from build123d import *

# Parameters (mm, degrees)
SKETCH1_W            = 81.28
SKETCH1_H            = 81.28
SKETCH1_W_2          = 76.2
SKETCH1_H_2          = 76.2
BOSS_EXTRUDE1_DEPTH  = 177.8
SKETCH2_W            = 2.54
SKETCH2_H            = 38.1
BOSS_EXTRUDE2_DEPTH  = 25.4
SKETCH3_W            = 2.54
SKETCH3_H            = 25.4
CUT_EXTRUDE1_DEPTH   = 212.720846399
BOSS_EXTRUDE3_DEPTH  = 12.7
BOSS_EXTRUDE4_DEPTH  = 12.7
SKETCH14_W           = 5.08
SKETCH14_H           = 25.4
BOSS_EXTRUDE6_DEPTH  = 76.2
CUT_EXTRUDE2_REACH   = 243.407
SKETCH16_W           = 23.13
SKETCH16_H           = 20.32
SKETCH22_R           = 2
CUT_EXTRUDE6_DEPTH   = 252.036309724
SKETCH28_W           = 35.399999812
SKETCH28_H           = 50.8
BOSS_EXTRUDE7_DEPTH  = 38.1
CUT_EXTRUDE8_REACH   = 246.574
SKETCH32_W           = 33.02
SKETCH32_H           = 30.319999812
CUT_EXTRUDE9_DEPTH   = 25.4
CUT_EXTRUDE13_REACH  = 245.27
SKETCH34_R           = 9.890000016
BOSS_EXTRUDE9_DEPTH  = 2.54
SKETCH38_W           = 2.54
SKETCH38_H           = 25.4
CUT_EXTRUDE15_DEPTH  = 63.5
CUT_EXTRUDE17_REACH  = 224.71
SKETCH40_R           = 2.999995
SKETCH41_R           = 3.77
SKETCH41_R_2         = 2.5
BOSS_EXTRUDE10_DEPTH = 5
BOSS_EXTRUDE11_START = 5
SKETCH42_R           = 3.77
SKETCH42_R_2         = 2.5
BOSS_EXTRUDE11_DEPTH = 5
SKETCH43_W           = 76.2
SKETCH43_H           = 76.2
CUT_EXTRUDE20_DEPTH  = 25.4
SKETCH44_W           = 174.6
SKETCH44_H           = 70
SKETCH44_R           = 1.5
BOSS_EXTRUDE12_DEPTH = 2.54
FILLET1_R            = 5.08
FILLET2_R            = 12.7
FILLET3_R            = 2.54
FILLET7_R            = 12.7
FILLET9_R            = 12.7
BOSS_EXTRUDE20_DEPTH = 88.9
CUT_EXTRUDE21_REACH  = 275.109
SKETCH54_R           = 2.5
FILLET11_R           = 2.54
FILLET12_R           = 2.54


with BuildPart() as part:
    # Sketch1 → Boss-Extrude1 (new body)
    with BuildSketch(Plane(origin=(0, 0, 0), x_dir=(1, 0, 0), z_dir=(0, 1, 0))):
        with Locations((40.64, 40.64)):
            Rectangle(SKETCH1_W, SKETCH1_H)
        with Locations((40.64, 40.64)):
            Rectangle(SKETCH1_W_2, SKETCH1_H_2, mode=Mode.SUBTRACT)
    extrude(amount=BOSS_EXTRUDE1_DEPTH)

    # Sketch2 → Boss-Extrude2 (add)
    with BuildSketch(Plane(origin=(0, 0, 0), x_dir=(0, 0, -1), z_dir=(1, 0, 0))):
        with Locations((64.77, 19.05)):
            Rectangle(SKETCH2_W, SKETCH2_H)
    extrude(amount=-BOSS_EXTRUDE2_DEPTH)

    # Sketch3 → Cut-Extrude1 (cut, through all)
    with BuildSketch(Plane.XY):
        with Locations((80.01, 12.7)):
            Rectangle(SKETCH3_W, SKETCH3_H)
    extrude(amount=-CUT_EXTRUDE1_DEPTH, mode=Mode.SUBTRACT)

    # Sketch7 → Boss-Extrude3 (add)
    with BuildSketch(Plane.XY):
        Polygon((81.28, 25.4), (106.68, 50.8), (81.28, 50.8), align=None)
    extrude(amount=-BOSS_EXTRUDE3_DEPTH)

    # Sketch10 → Boss-Extrude4 (add)
    with BuildSketch(Plane(origin=(0, 0, -81.28), x_dir=(-1, 0, 0), z_dir=(0, 0, -1))):
        Polygon((-81.28, 25.4), (-81.28, 50.8), (-106.68, 50.8), align=None)
    extrude(amount=-BOSS_EXTRUDE4_DEPTH)

    # Sketch14 → Boss-Extrude6 (add)
    with BuildSketch(Plane(origin=(81.28, 0, 0), x_dir=(0, 0, -1), z_dir=(1, 0, 0))):
        with Locations((40.64, 38.1)):
            Rectangle(SKETCH14_W, SKETCH14_H)
    extrude(amount=BOSS_EXTRUDE6_DEPTH)

    # Sketch16 → Cut-Extrude2 (cut, up to next)
    with BuildSketch(Plane.XY.offset(-38.1), mode=Mode.PRIVATE) as cut_extrude2_sk1:
        with Locations((129.405, 40.64)):
            Rectangle(SKETCH16_W, SKETCH16_H)
    cut_extrude2_tool1 = extrude(cut_extrude2_sk1.sketch, amount=-CUT_EXTRUDE2_REACH, mode=Mode.PRIVATE) & part.part
    add(cut_extrude2_tool1.solids().sort_by_distance((129.405, 40.64, -38.1))[0], mode=Mode.SUBTRACT)

    # Sketch22 → Cut-Extrude6 (cut, through all)
    with BuildSketch(Plane.XY):
        with Locations((93.98, 45.72)):
            Circle(SKETCH22_R)
    extrude(amount=-CUT_EXTRUDE6_DEPTH, mode=Mode.SUBTRACT)

    # Sketch28 → Boss-Extrude7 (add)
    with BuildSketch(Plane(origin=(81.28, 0, 0), x_dir=(0, 0, -1), z_dir=(1, 0, 0))):
        with Locations((40.64, 152.4)):
            Rectangle(SKETCH28_W, SKETCH28_H)
    extrude(amount=BOSS_EXTRUDE7_DEPTH)

    # Sketch30 → Cut-Extrude8 (cut, up to next)
    with BuildSketch(Plane.XY.offset(-22.940000094), mode=Mode.PRIVATE) as cut_extrude8_sk1:
        Polygon((81.28, 127), (119.38, 127), (119.38, 152.4), align=None)
    cut_extrude8_tool1 = extrude(cut_extrude8_sk1.sketch, amount=-CUT_EXTRUDE8_REACH, mode=Mode.PRIVATE) & part.part
    add(cut_extrude8_tool1.solids().sort_by_distance((106.68, 135.466667, -22.94))[0], mode=Mode.SUBTRACT)

    # Sketch32 → Cut-Extrude9 (cut)
    with BuildSketch(Plane(origin=(0, 177.8, 0), x_dir=(1, 0, 0), z_dir=(0, 1, 0))):
        with Locations((100.33, 40.64)):
            Rectangle(SKETCH32_W, SKETCH32_H)
    extrude(amount=-CUT_EXTRUDE9_DEPTH, mode=Mode.SUBTRACT)

    # Cut-Extrude13: up to this face of the body (flat: up to its plane)
    cut_extrude13_end = Plane(part.part.faces().sort_by_distance((78.74, 101.6, -40.64))[0])
    # Sketch34 → Cut-Extrude13 (cut, up to the picked face)
    with BuildSketch(Plane(origin=(119.38, 0, 0), x_dir=(0, 0, -1), z_dir=(1, 0, 0)), mode=Mode.PRIVATE) as cut_extrude13_sk1:
        with Locations(Location((40.593000094, 165.1, 0), (0, 0, 180))):
            Circle(SKETCH34_R)
    cut_extrude13_tool1 = split(extrude(cut_extrude13_sk1.sketch, amount=-CUT_EXTRUDE13_REACH, mode=Mode.PRIVATE), bisect_by=cut_extrude13_end, keep=Keep.BOTH, mode=Mode.PRIVATE)
    add(cut_extrude13_tool1.solids().sort_by(Axis((119.38, 165.1, -40.593), (-1, 0, 0)))[0], mode=Mode.SUBTRACT)

    # Sketch37 → Boss-Extrude9 (add)
    with BuildSketch(Plane.XY.offset(-63.5)):
        Polygon((-25.4, 38.1), (0, 38.1), (0, 52.764696837), align=None)
    extrude(amount=-BOSS_EXTRUDE9_DEPTH)

    # Sketch38 → Cut-Extrude15 (cut)
    with BuildSketch(Plane.XY):
        with Locations((1.27, 12.7)):
            Rectangle(SKETCH38_W, SKETCH38_H)
    extrude(amount=-CUT_EXTRUDE15_DEPTH, mode=Mode.SUBTRACT)

    # Cut-Extrude17: up to this face of the body (flat: up to its plane)
    cut_extrude17_end = Plane(part.part.faces().sort_by_distance((0, 99.23335202, -41.514066738))[0])
    # Sketch40 → Cut-Extrude17 (cut, up to the picked face)
    with BuildSketch(Plane(origin=(81.28, 0, 0), x_dir=(0, 0, -1), z_dir=(1, 0, 0)), mode=Mode.PRIVATE) as cut_extrude17_sk1:
        with Locations((19.05, 101.6)):
            Circle(SKETCH40_R)
    cut_extrude17_tool1 = split(extrude(cut_extrude17_sk1.sketch, amount=-CUT_EXTRUDE17_REACH, mode=Mode.PRIVATE), bisect_by=cut_extrude17_end, keep=Keep.BOTH, mode=Mode.PRIVATE)
    # Sketch40 → Cut-Extrude17 (cut, up to the picked face)
    with BuildSketch(Plane(origin=(81.28, 0, 0), x_dir=(0, 0, -1), z_dir=(1, 0, 0)), mode=Mode.PRIVATE) as cut_extrude17_sk2:
        with Locations((62.23, 101.6)):
            Circle(SKETCH40_R)
    cut_extrude17_tool2 = split(extrude(cut_extrude17_sk2.sketch, amount=-CUT_EXTRUDE17_REACH, mode=Mode.PRIVATE), bisect_by=cut_extrude17_end, keep=Keep.BOTH, mode=Mode.PRIVATE)
    add(cut_extrude17_tool1.solids().sort_by(Axis((81.28, 101.6, -19.05), (-1, 0, 0)))[0], mode=Mode.SUBTRACT)
    add(cut_extrude17_tool2.solids().sort_by(Axis((81.28, 101.6, -62.23), (-1, 0, 0)))[0], mode=Mode.SUBTRACT)

    # Sketch41 → Boss-Extrude10 (add)
    # profile 1 of 2: a face of its own
    with BuildSketch(Plane(origin=(81.28, 0, 0), x_dir=(0, 0, -1), z_dir=(1, 0, 0))):
        with Locations(Location((19.05, 101.6, 0), (0, 0, 180))):
            Circle(SKETCH41_R)
        with Locations((19.05, 101.6)):
            Circle(SKETCH41_R_2, mode=Mode.SUBTRACT)
    # profile 2 of 2: a face of its own
    with BuildSketch(Plane(origin=(81.28, 0, 0), x_dir=(0, 0, -1), z_dir=(1, 0, 0))):
        with Locations(Location((62.23, 101.6, 0), (0, 0, 180))):
            Circle(SKETCH41_R)
        with Locations((62.23, 101.6)):
            Circle(SKETCH41_R_2, mode=Mode.SUBTRACT)
    extrude(amount=BOSS_EXTRUDE10_DEPTH)

    # Sketch42 → Boss-Extrude11 (add)
    # profile 1 of 2: a face of its own
    with BuildSketch(Plane.ZY.offset(BOSS_EXTRUDE11_START)):
        with Locations((-62.23, 101.6)):
            Circle(SKETCH42_R)
        with Locations(Location((-62.23, 101.6, 0), (0, 0, 180))):
            Circle(SKETCH42_R_2, mode=Mode.SUBTRACT)
    # profile 2 of 2: a face of its own
    with BuildSketch(Plane.ZY.offset(BOSS_EXTRUDE11_START)):
        with Locations((-19.05, 101.6)):
            Circle(SKETCH42_R)
        with Locations(Location((-19.05, 101.6, 0), (0, 0, 180))):
            Circle(SKETCH42_R_2, mode=Mode.SUBTRACT)
    extrude(amount=-BOSS_EXTRUDE11_DEPTH)

    # Sketch43 → Cut-Extrude20 (cut)
    with BuildSketch(Plane(origin=(0, 177.8, 0), x_dir=(1, 0, 0), z_dir=(0, 1, 0))):
        Polygon((83.82, 58.339999906), (83.82, 22.940000094), (81.28, 22.940000094), (81.28, 0), (0, 0), (0, 81.28), (81.28, 81.28), (81.28, 58.339999906), align=None)
        with Locations((40.64, 40.64)):
            Rectangle(SKETCH43_W, SKETCH43_H, mode=Mode.SUBTRACT)
    extrude(amount=-CUT_EXTRUDE20_DEPTH, mode=Mode.SUBTRACT)

    # Sketch44 → Boss-Extrude12 (add)
    with BuildSketch(Plane.XY):
        with Locations((87.3, 85.8)):
            Rectangle(SKETCH44_W, SKETCH44_H)
        with Locations((140.97, 115.8)):
            Circle(SKETCH44_R, mode=Mode.SUBTRACT)
        with Locations((140.97, 55.8)):
            Circle(SKETCH44_R, mode=Mode.SUBTRACT)
    extrude(amount=-BOSS_EXTRUDE12_DEPTH)

    # Fillet1
    fillet1_edges = [part.edges().sort_by_distance(p)[0] for p in [
        (106.68, 50.8, -7.62),
        (106.68, 50.8, -74.93),
    ]]
    fillet(fillet1_edges, radius=FILLET1_R)

    # Fillet2
    fillet2_edges = [part.edges().sort_by_distance(p)[0] for p in [
        (174.6, 120.8, -1.27),
        (174.6, 50.8, -1.27),
    ]]
    fillet(fillet2_edges, radius=FILLET2_R)

    # Fillet3
    fillet3_edges = [part.edges().sort_by_distance(p)[0] for p in [
        (157.48, 50.8, -40.64),
        (157.48, 25.4, -40.64),
    ]]
    fillet(fillet3_edges, radius=FILLET3_R)

    # Fillet7
    fillet7_edges = [part.edges().sort_by_distance(p)[0] for p in [
        (-25.4, 38.1, -64.77),
    ]]
    fillet(fillet7_edges, radius=FILLET7_R)

    # Fillet9
    fillet9_edges = [part.edges().sort_by_distance(p)[0] for p in [
        (83.82, 177.8, -24.210000094),
        (83.82, 177.8, -57.069999906),
    ]]
    fillet(fillet9_edges, radius=FILLET9_R)

    # Sketch53 → Boss-Extrude20 (add)
    with BuildSketch(Plane(origin=(0, 0, 0), x_dir=(-1, 0, 0), z_dir=(0, -1, 0))):
        Polygon((-35.659105782, 81.28), (-35.659105782, 78.74), (-45.72, 78.74), (-45.72, 111.76), (-15.24, 111.76), (-15.24, 106.68), (-40.64, 106.68), (-40.64, 81.28), align=None)
    extrude(amount=-BOSS_EXTRUDE20_DEPTH)

    # Sketch54 → Cut-Extrude21 (cut, up to next)
    with BuildSketch(Plane(origin=(0, 0, -111.76), x_dir=(-1, 0, 0), z_dir=(0, 0, -1)), mode=Mode.PRIVATE) as cut_extrude21_sk1:
        with Locations((-30.48, 76.2)):
            Circle(SKETCH54_R)
    cut_extrude21_tool1 = extrude(cut_extrude21_sk1.sketch, amount=-CUT_EXTRUDE21_REACH, mode=Mode.PRIVATE) & part.part
    # Sketch54 → Cut-Extrude21 (cut, up to next)
    with BuildSketch(Plane(origin=(0, 0, -111.76), x_dir=(-1, 0, 0), z_dir=(0, 0, -1)), mode=Mode.PRIVATE) as cut_extrude21_sk2:
        with Locations((-30.48, 44.45)):
            Circle(SKETCH54_R)
    cut_extrude21_tool2 = extrude(cut_extrude21_sk2.sketch, amount=-CUT_EXTRUDE21_REACH, mode=Mode.PRIVATE) & part.part
    # Sketch54 → Cut-Extrude21 (cut, up to next)
    with BuildSketch(Plane(origin=(0, 0, -111.76), x_dir=(-1, 0, 0), z_dir=(0, 0, -1)), mode=Mode.PRIVATE) as cut_extrude21_sk3:
        with Locations((-30.48, 12.7)):
            Circle(SKETCH54_R)
    cut_extrude21_tool3 = extrude(cut_extrude21_sk3.sketch, amount=-CUT_EXTRUDE21_REACH, mode=Mode.PRIVATE) & part.part
    add(cut_extrude21_tool1.solids().sort_by_distance((30.48, 76.2, -111.76))[0], mode=Mode.SUBTRACT)
    add(cut_extrude21_tool2.solids().sort_by_distance((30.48, 44.45, -111.76))[0], mode=Mode.SUBTRACT)
    add(cut_extrude21_tool3.solids().sort_by_distance((30.48, 12.7, -111.76))[0], mode=Mode.SUBTRACT)

    # Fillet11
    fillet11_edges = [part.edges().sort_by_distance(p)[0] for p in [
        (15.24, 0, -109.22),
        (15.24, 88.9, -109.22),
        (15.24, 44.45, -111.76),
        (15.24, 44.45, -106.68),
    ]]
    fillet(fillet11_edges, radius=FILLET11_R - 0.0001)  # a hair under: the kernel refuses the full size

    # Fillet12
    fillet12_edges = [part.edges().sort_by_distance(p)[0] for p in [
        (81.28, 136.6, 0),
        (81.28, 101.6, -81.28),
        (0, 76.2, -81.28),
        (0, 88.9, 0),
    ]]
    fillet(fillet12_edges, radius=FILLET12_R)


solid = part.part
Design review of the part built by this model. Coordinates are the model's own, in mm. A direction names the side the tool comes from. Give positions to 0.01 mm unless a question says otherwise; leave off trailing zeros. Write each loop counter-clockwise with the first axis right and the second up, starting at its lowest first coordinate (ties: lowest second). Pieces come first, ordered by that corner, then holes. Notation, with made-up numbers: M -7,17 L 15,17 A15 ccw 15,28 Z; hole C 31,33 d1. An arc over 180 degrees is marked long. Return JSON: item names as keys, results as strings. Group by question number.
Item 1: Take a section at B-B (y = 12.7). Count the separate pieces of the cut face and the enclosed holes in it, plus the area to 3 significant figures.
Item 2: Take a section at C-C (x = 30.48). Give the boundary of the cut face in (y, z).
Item 3: Wall thickness on line 1 along X through (y, z) = (116, -14.5); line 2 along Y through (x, z) = (-2.5, -19.05); line 3 along Z through (x, y) = (1, 101): over which ranges is each line inside the solid? List them lowest first.
Item 4: Clearance check with flat-ended pins moving along their axes: pin 1 Ø3 at (y, z) = (51, -36) entering from +X; pin 2 Ø3 at (y, z) = (15.5, -1) entering from -X; pin 3 Ø6.5 at (y, z) = (101.6, -19.05) entering from +X; pin 4 Ø3.5 at (x, y) = (93.98, 45.72) entering from -Z. State where each tip first meets the part, or that it passes through.
Item 5: Tool access review of faces 1 (the flat face through (45.72, 44, -96)), 2 (the cylindrical face through (1.29, 102.5, -65.09)), 3 (the cylindrical face through (99.14, 47.59, -7.69)), 4 (the flat face through (2.54, 92, -40)): name each direction out of +Z, -Z, +X, -X, +Y, -Y from which nothing blocks a thin tool from reaching the whole face with its end or side.
Item 6: The part is to be moulded in two halves that separate along Y. For faces 5 (the cylindrical face through (83.74, 104.08, -18.72)), 6 (the flat face through (127, 91, -2.54)), 7 (the flat face through (117, 177.8, -42)), say which applies: pulls with the +Y half, pulls with the -Y half, needs draft (parallel to the pull), parting line crosses it, or undercut.
Item 7: Take a section at A-A (z = -71.5). Give the boundary of the cut face in (x, y), plus the area to 3 significant figures.
Return value:
{
 "1": {"separate pieces": "3", "enclosed holes": "0", "area": "751 mm2"},
 "2": {"outline": "M 0,-111.76 L 10.2,-111.76 L 10.2,-106.68 L 0,-106.68 Z; M 0,-81.28 L 152.4,-81.28 L 152.4,-78.74 L 0,-78.74 Z; M 0,-2.54 L 152.4,-2.54 L 152.4,0 L 0,0 Z; M 15.2,-111.76 L 41.95,-111.76 L 41.95,-106.68 L 15.2,-106.68 Z; M 46.95,-111.76 L 73.7,-111.76 L 73.7,-106.68 L 46.95,-106.68 Z; M 78.7,-111.76 L 88.9,-111.76 L 88.9,-106.68 L 78.7,-106.68 Z"},
 "3": {"line 1": "x = 0 to 2.54, 78.74 to 81.28", "line 2": "y = 97.83 to 99.1, 104.1 to 105.37", "line 3": "z = -80.76 to -65.17, -59.29 to -21.99, -16.11 to -0.52"},
 "4": {"pin 1": "stops at x = 81.28", "pin 2": "stops at x = 2.54", "pin 3": "stops at x = 86.28", "pin 4": "passes through"},
 "5": {"face 1": "-Z, +X, +Y, -Y", "face 2": "none", "face 3": "+X", "face 4": "+Y, -Y"},
 "6": {"face 5": "undercut", "face 6": "needs draft", "face 7": "pulls with the +Y half"},
 "7": {"outline": "M 0,0 L 2.54,0 L 2.54,152.4 L 0,152.4 Z; M 78.74,25.4 L 81.28,25.4 L 98.01,42.13 A5.08 ccw 94.42,50.8 L 81.28,50.8 L 81.28,152.4 L 78.74,152.4 Z; hole C 93.98,45.72 d4", "area": "988 mm2"}
}
